Autodesk Inventor part; units mm, degrees
ref_plane "YZ Plane" through (0, 0, 0) normal (1, 0, 0) x (0, 1, 0)
ref_plane "XZ Plane" through (0, 0, 0) normal (0, 1, 0) x (-1, 0, 0)
ref_plane "XY Plane" through (0, 0, 0) normal (0, 0, 1) x (1, 0, 0)
sketch "Boceto1" plane through (0, 0, 0) normal (0, 1, 0) x (-1, 0, 0)
  circle A0 centre (0, 0) radius 7.9375
  dimension "d0" = 15.875
extrude "Extrusión1" add sketch "Boceto1" along normal blind 165.1
sketch "Boceto2" plane through (0, 0, 0) normal (0, -1, 0) x (1, 0, 0)
  circle A0 centre (0, 0) radius 9.525
  dimension "d3" = 19.05
extrude "Extrusión2" add sketch "Boceto2" against normal blind 12.7
sketch "Boceto3" plane through (0, 165.1, 0) normal (0, 1, 0) x (1, 0, 0)
  circle A0 centre (0, 0) radius 9.525
  dimension "d6" = 19.05
extrude "Extrusión3" add sketch "Boceto3" against normal blind 25.4
chamfer "Chaflán1" distance 1.5875 angle 45 1 edges at (-9.525, 165.1, 0) measured on face at (0.831, 165.1, 0.7598)
sketch "Boceto4" plane through (0, 0, 0) normal (1, 0, 0) x (0, 1, 0)
  line L0 (165.1, 7.9375) -> (165.1, -7.9375)
  line L1 (165.1, 0) -> (139.7, 0)
  line L2 (139.7, 9.525) -> (139.7, -9.525)
  circle A0 centre (152.4, 0) radius 4.7625
  point P0 (0, 0)
  dimension "d12" = 9.525
extrude "Extrusión4" cut sketch "Boceto4" along normal mid plane 25.4
properties part number "Pieza7-Tarea1"
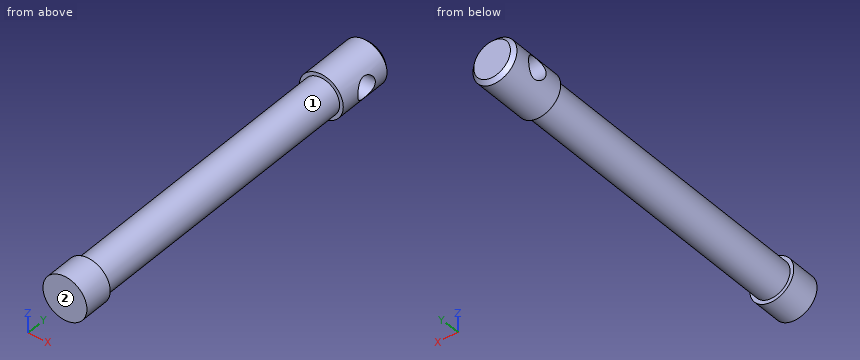
Input: part model. Units: mm. Frame: model coordinates. Face numbers are marked on the shaded views. A direction names the side the tool comes from. Give positions to 0.01 mm unless a question says otherwise; leave off trailing zeros. Order: outer loops, then holes, each group sorted by start corner. A loop starts at its lowest first (then second) coordinate and runs counter-clockwise, first axis right, second up. Notation, with made-up numbers: (-26, -35) - (-16, -35) arc R29 ccw to (-16, 0) - close; hole circle Ø1 at (44.25, 16.5). An arc over 180 degrees is marked (long way). Put each result on its own line as item: value.
Item 1: Ray query, L1, parallel to Y at x = -4.75, z = 0; L2, parallel to Z at x = -0.5, y = 152.4; L3, parallel to Y at x = 0.25, z = 1.5. Return the intervals inside material, ascending. Write a range as from..to.
Found:
L1: y = 0..147.64, 157.16..165.1
L2: z = -9.51..-4.76, 4.76..9.51
L3: y = 0..147.88, 156.92..165.1
Item 2: Access query for the marked faces 1 and 2. Directions: +Z, -Z, +X, -X, +Y, -Y. A direction counts if a zero-diameter tool reaches every point of the face in a straight line with its end or side. Return the directions, or none.
Found:
face 1: none
face 2: +Z, -Z, +X, -X, -Y
Item 3: Section query A-A, the plane z = 0. Return loops of the section in (x, y) (1 decimal).
Found:
outline: (-9.5, 0) - (9.5, 0) - (9.5, 12.7) - (7.9, 12.7) - (7.9, 139.7) - (9.5, 139.7) - (9.5, 147.6) - (-9.5, 147.6) - (-9.5, 139.7) - (-7.9, 139.7) - (-7.9, 12.7) - (-9.5, 12.7) - close; (-9.5, 157.2) - (9.5, 157.2) - (9.5, 163.5) - (7.9, 165.1) - (-7.9, 165.1) - (-9.5, 163.5) - close
Item 4: Section query B-B, the plane x = 0. Return loops of the section in (y, z) (1 decimal).
Found:
outline: (0, -9.5) - (12.7, -9.5) - (12.7, -7.9) - (139.7, -7.9) - (139.7, -9.5) - (163.5, -9.5) - (165.1, -7.9) - (165.1, 7.9) - (163.5, 9.5) - (139.7, 9.5) - (139.7, 7.9) - (12.7, 7.9) - (12.7, 9.5) - (0, 9.5) - close; hole circle Ø9.5 at (152.4, 0)
Item 5: Contact query for flat-ended pins moving along their axis: pin 1 (3 mm diameter, centred on x = -6.5, y = 98, fed in from +Z); pin 2 (6 mm diameter, centred on y = 19, z = 5, fed in from +X); pin 3 (6 mm diameter, centred on x = -2, y = 72.5, fed in from +Z); pin 4 (8.5 mm diameter, centred on y = 152.4, z = 0, fed in from +X). Output: stop coordinate, or through.
Found:
pin 1: stops at z = 6.16
pin 2: stops at x = 7.68
pin 3: stops at z = 7.94
pin 4: passes through
Item 6: Section query D-D, the plane y = 48. Return loops of the section in (x, z) (1 decimal), then the cut area to 3 significant figures.
Found:
outline: circle Ø15.9 at (0, 0)
area: 198 mm^2
